Could you check a few things on this drawing? It's one solid part, dimensions in mm from its lowest x, y, z. Round coordinates to 2 decimals unless told otherwise and drop trailing zeros. Write each loop counter-clockwise with the first axis right and the second up, starting at its lowest first coordinate (ties: lowest second). Pieces come first, ordered by that corner, then holes. Notation, with made-up numbers: (42, 22.5) -> (50, 22.5) arc R17 cw to (50, 40.5) -> close; hole circle Ø8 at (-22.75, 79.5). An arc over 180 degrees is marked (long way). Answer in a Markdown table with one row per item. Add a question column.
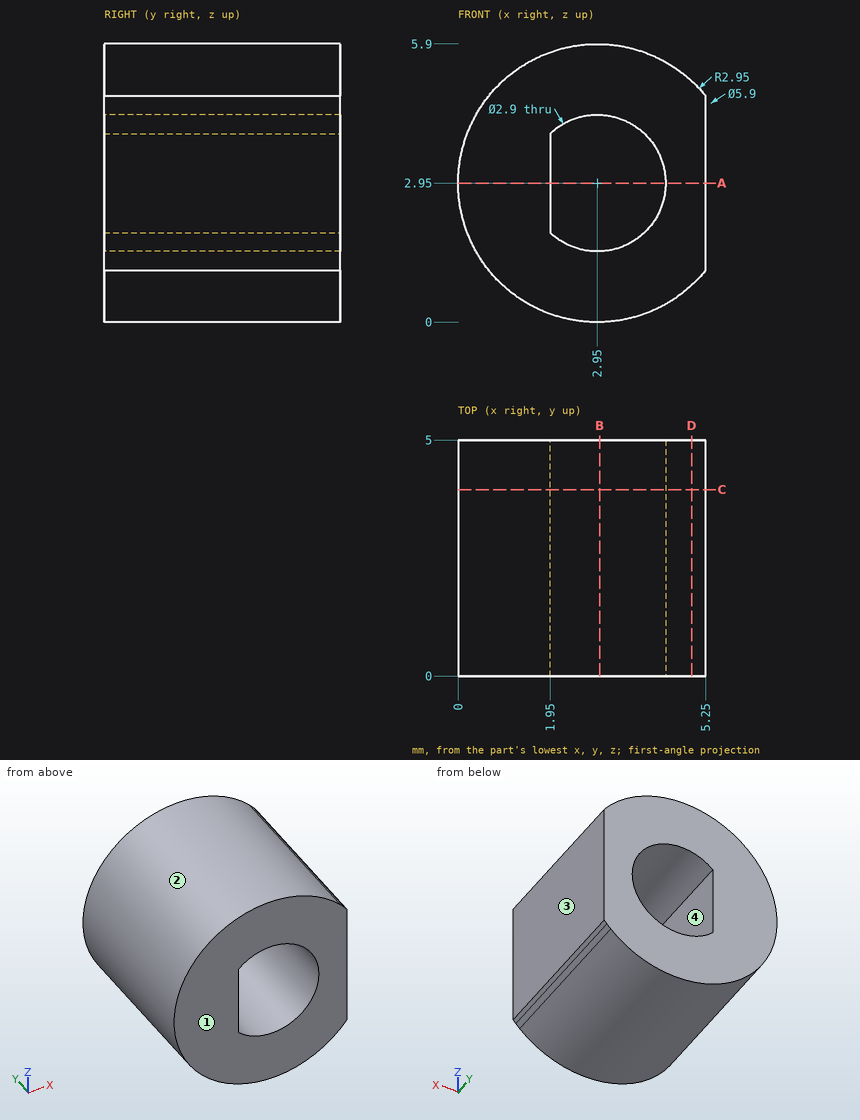
Item 1: If we section it at A-A on z = 2.95: Please give me the cut outline in (x, y), then the cut area to 3 significant figures.
Item 2: If we section it at D-D on x = 4.95: Please give me the cut outline in (y, z).
Item 3: If we mould it in two halves opening along X, with no side actions, what happens to the marked faces 1, 2, 3 and 4? For each: pulls with the +X half, pulls with the -X half, needs draft (parallel to the pull), parting line crosses it, or undercut.
Item 4: If we section it at B-B on x = 3: Please give me the cut outline in (y, z).
Item 5: If we section it at C-C on y = 3.95: Please give me the cut outline in (x, z).
Item 6: I need wall thicknesses on line 1 along Z through (x, y) = (2.95, 1.4); line 2 along X through (y, z) = (2.05, 3.4); line 3 along X through (y, z) = (2.6, 2.2). Which ranges of each line are inside material? Lowest first, please. Write a range as from..to.
Results list:
| question | item | result |
|---|---|---|
| 1 | outline | (0, 0) -> (1.95, 0) -> (1.95, 5) -> (0, 5) -> close; (4.4, 0) -> (5.25, 0) -> (5.25, 5) -> (4.4, 5) -> close |
| 1 | area | 14.0 mm² |
| 2 | outline | (0, 0.78) -> (5, 0.78) -> (5, 5.12) -> (0, 5.12) -> close |
| 3 | face 1 | needs draft |
| 3 | face 2 | parting line crosses it |
| 3 | face 3 | pulls with the +X half |
| 3 | face 4 | undercut |
| 4 | outline | (0, 0) -> (5, 0) -> (5, 1.5) -> (0, 1.5) -> close; (0, 4.4) -> (5, 4.4) -> (5, 5.9) -> (0, 5.9) -> close |
| 5 | outline | (5.05, 0.88) arc R2.95 ccw to (5.17, 1) arc R2.95 ccw to (5.25, 1.1) -> (5.25, 4.8) arc R2.95 ccw (long way) to start; hole (1.95, 1.9) arc R1.45 ccw (long way) to (1.95, 4) -> close |
| 6 | line 1 | 0..1.5, 4.4..5.9 |
| 6 | line 2 | 0.03..1.95, 4.33..5.25 |
| 6 | line 3 | 0.1..1.95, 4.19..5.25 |
